```python
from build123d import *

# Parameters (mm, degrees)
F1_R     = 67.5
F1_R_2   = 2.5
F1_R_3   = 17.5
F2_DEPTH = 6
F0_R     = 17.5
F3_DEPTH = 12


with BuildPart() as f2:
    # F1 (on face) → F2 (new body)
    with BuildSketch(Plane.XY):
        Circle(F1_R)
        with Locations((-21.950199, -54.490424)):
            Circle(F1_R_2, mode=Mode.SUBTRACT)
        with Locations((-7.146533, -61.046224)):
            Circle(F1_R_2, mode=Mode.SUBTRACT)
        with Locations((-7.802248, -45.019042)):
            Circle(F1_R_2, mode=Mode.SUBTRACT)
        with Locations((-47.73964, -18.328615)):
            Circle(F1_R_2, mode=Mode.SUBTRACT)
        with Locations((-56.234829, -9.563138)):
            Circle(F1_R_2, mode=Mode.SUBTRACT)
        with Locations((9.563138, -56.234829)):
            Circle(F1_R_2, mode=Mode.SUBTRACT)
        with Locations((18.328615, -47.73964)):
            Circle(F1_R_2, mode=Mode.SUBTRACT)
        with BuildLine():
            Line((-28.752191, -35.313599), (-4.075158, -17.97025))
            ThreePointArc((-4.075158, -17.97025), (-3.528223, -17.69964), (-2.925146, -17.606548))
            Line((-2.925146, -17.606548), (0, -17.606548))
            Line((0, -17.606548), (2.925146, -17.606548))
            ThreePointArc((2.925146, -17.606548), (3.528223, -17.69964), (4.075158, -17.97025))
            Line((4.075158, -17.97025), (28.752191, -35.313599))
            ThreePointArc((28.752191, -35.313599), (29.509087, -37.552974), (27.602179, -38.949897))
            Line((27.602179, -38.949897), (0, -38.949897))
            Line((0, -38.949897), (-27.602179, -38.949897))
            ThreePointArc((-27.602179, -38.949897), (-29.509087, -37.552974), (-28.752191, -35.313599))
        make_face(mode=Mode.SUBTRACT)
        with Locations((54.490424, -21.950199)):
            Circle(F1_R_2, mode=Mode.SUBTRACT)
        with Locations((45.019042, -7.802248)):
            Circle(F1_R_2, mode=Mode.SUBTRACT)
        with Locations((61.046224, -7.146533)):
            Circle(F1_R_2, mode=Mode.SUBTRACT)
        with Locations((-61.046224, 7.146533)):
            Circle(F1_R_2, mode=Mode.SUBTRACT)
        with Locations((-45.019042, 7.802248)):
            Circle(F1_R_2, mode=Mode.SUBTRACT)
        with Locations((-54.490424, 21.950199)):
            Circle(F1_R_2, mode=Mode.SUBTRACT)
        with BuildLine():
            Line((-35.313599, 28.752191), (-17.97025, 4.075158))
            ThreePointArc((-17.97025, 4.075158), (-17.69964, 3.528223), (-17.606548, 2.925146))
            Line((-17.606548, 2.925146), (-17.606548, 0))
            Line((-17.606548, 0), (-17.606548, -2.925146))
            ThreePointArc((-17.606548, -2.925146), (-17.69964, -3.528223), (-17.97025, -4.075158))
            Line((-17.97025, -4.075158), (-35.313599, -28.752191))
            ThreePointArc((-35.313599, -28.752191), (-37.552974, -29.509087), (-38.949897, -27.602179))
            Line((-38.949897, -27.602179), (-38.949897, 0))
            Line((-38.949897, 0), (-38.949897, 27.602179))
            ThreePointArc((-38.949897, 27.602179), (-37.552974, 29.509087), (-35.313599, 28.752191))
        make_face(mode=Mode.SUBTRACT)
        with Locations((-18.328615, 47.73964)):
            Circle(F1_R_2, mode=Mode.SUBTRACT)
        with Locations((-9.563138, 56.234829)):
            Circle(F1_R_2, mode=Mode.SUBTRACT)
        Circle(F1_R_3, mode=Mode.SUBTRACT)
        with BuildLine():
            Line((35.313599, -28.752191), (17.97025, -4.075158))
            ThreePointArc((17.97025, -4.075158), (17.69964, -3.528223), (17.606548, -2.925146))
            Line((17.606548, -2.925146), (17.606548, 0))
            Line((17.606548, 0), (17.606548, 2.925146))
            ThreePointArc((17.606548, 2.925146), (17.69964, 3.528223), (17.97025, 4.075158))
            Line((17.97025, 4.075158), (35.313599, 28.752191))
            ThreePointArc((35.313599, 28.752191), (37.552974, 29.509087), (38.949897, 27.602179))
            Line((38.949897, 27.602179), (38.949897, 0))
            Line((38.949897, 0), (38.949897, -27.602179))
            ThreePointArc((38.949897, -27.602179), (37.552974, -29.509087), (35.313599, -28.752191))
        make_face(mode=Mode.SUBTRACT)
        with BuildLine():
            ThreePointArc((27.602179, 38.949897), (29.509087, 37.552974), (28.752191, 35.313599))
            Line((28.752191, 35.313599), (4.075158, 17.97025))
            ThreePointArc((4.075158, 17.97025), (3.528223, 17.69964), (2.925146, 17.606548))
            Line((2.925146, 17.606548), (0, 17.606548))
            Line((0, 17.606548), (-2.925146, 17.606548))
            ThreePointArc((-2.925146, 17.606548), (-3.528223, 17.69964), (-4.075158, 17.97025))
            Line((-4.075158, 17.97025), (-28.752191, 35.313599))
            ThreePointArc((-28.752191, 35.313599), (-29.509087, 37.552974), (-27.602179, 38.949897))
            Line((-27.602179, 38.949897), (0, 38.949897))
            Line((0, 38.949897), (27.602179, 38.949897))
        make_face(mode=Mode.SUBTRACT)
        with Locations((56.234829, 9.563138)):
            Circle(F1_R_2, mode=Mode.SUBTRACT)
        with Locations((47.73964, 18.328615)):
            Circle(F1_R_2, mode=Mode.SUBTRACT)
        with Locations((7.802248, 45.019042)):
            Circle(F1_R_2, mode=Mode.SUBTRACT)
        with Locations((7.146533, 61.046224)):
            Circle(F1_R_2, mode=Mode.SUBTRACT)
        with Locations((21.950199, 54.490424)):
            Circle(F1_R_2, mode=Mode.SUBTRACT)
    extrude(amount=F2_DEPTH)

    # F0 (on Top) → F3 (join)
    with BuildSketch(Plane.XY):
        Circle(F0_R)
    extrude(amount=F3_DEPTH)


solid = f2.part
```
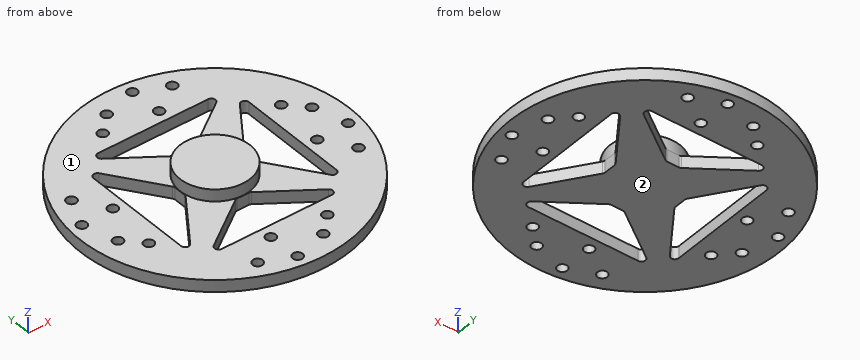
Model file for the job. Use its own axes, mm. Face numbers are marked on the shaded views. A direction names the side the tool comes from. Give positions to 0.01 mm unless a question says otherwise; leave off trailing zeros. Loops run counter-clockwise (first coordinate to the right, second up) from the corner with the lowest first, then second, coordinate; pieces in that order, holes last. Notation, with made-up numbers: (-15, 16.5) -> (37, 16.5) arc R35 cw to (37, 52.5) -> close; hole circle Ø4 at (42, 21.25). An arc over 180 degrees is marked (long way). Write each question's results on one line, items separated by ' | '.
(1) Cut at C-C on z = 8. List the corners of the cut face in (x, y).
Geometry results:
outline: circle Ø35 at (0, 0)
(2) Tool access for the marked faces 1 and 2: list every direction of +Z, -Z, +X, -X, +Y, -Y with a clear straight run to the whole face (end or side of a thin tool).
Geometry results:
face 1: +Z | face 2: -Z, +X, -X, +Y, -Y
(3) Probe line 1 along X through (y, z) = (-18, 0.75); line 2 along Y through (x, z) = (-11.5, 4.5); line 3 along X through (y, z) = (7.5, 2.25). List the from-to ranges inside material, lowest first.
Geometry results:
line 1: x = -65.06 to -50.22, -45.26 to -38.95, -27.76 to -4.12, 4.12 to 27.76, 38.95 to 65.06 | line 2: y = -66.51 to -38.95, -23.19 to 23.19, 38.95 to 54.65, 57.82 to 66.51 | line 3: x = -67.08 to -63.52, -58.57 to -47.5, -42.54 to -38.95, -20.38 to 20.38, 38.95 to 54.82, 57.65 to 67.08
(4) Flat gauge pins, fed straight in: pin 1 Ø4 at (y, z) = (-45, 1.5) entering from +X; pin 2 Ø6 at (x, y) = (-53.5, 39.5) entering from +Z; pin 3 Ø1.8 at (x, z) = (1.5, 2) entering from +Y. Where does each tip first touch, or does it go through?
Geometry results:
pin 1: stops at x = 52.03 | pin 2: stops at z = 6 | pin 3: stops at y = 67.5
(5) Cut at A-A on x = 0. List the corners of the cut face in (y, z), and give its area (3 significant figures).
Geometry results:
outline: (-67.5, 0) -> (-38.95, 0) -> (-38.95, 6) -> (-67.5, 6) -> close; (-17.61, 0) -> (17.61, 0) -> (17.61, 6) -> (17.5, 6) -> (17.5, 12) -> (-17.5, 12) -> (-17.5, 6) -> (-17.61, 6) -> close; (38.95, 0) -> (67.5, 0) -> (67.5, 6) -> (38.95, 6) -> close | area: 764 mm²
